Could you check a few things on this model? Use its own coordinates, in mm. Coordinates: 2 decimals unless noted, no trailing zeros. Loops run counter-clockwise (first coordinate to the right, second up) from the corner with the lowest first, then second, coordinate; pieces in that order, holes last.
1) Imagine slicing it at D-D on z = 0.4. Give the number of separate pieces and of enclosed holes in the cut face, plus the area to 3 significant figures.
2) Imagine slicing it at B-B on y = 26. Please give me the cut outline in (x, z).
3) Imagine slicing it at C-C on x = 5. Please give me the cut outline in (y, z).
4) Imagine slicing it at A-A on x = 32. Please give me the cut outline in (y, z).
5) If I drill on line 1 along X through (y, z) = (-3, 0.75); line 2 along Y through (x, z) = (-18, 0.9); line 3 along Y through (x, z) = (4, 0.25), over which ranges is the centre line in solid material (lowest first)?
6) Will these pins go through, and if not, where does the flat tip stop? P1, Ø0.6, axis at x = 22.5, z = 1, coming from the -Y side; P2, Ø0.6, axis at x = 17.5, z = 1.5, coming from the +Y side; P3, Ø1, axis at x = 17.5, z = 1.5, coming from the -Y side; P4, Ø3.5, axis at x = 32.63, y = 15.21, coming from the +Z side.
```python
from build123d import *

# Parameters (mm, degrees)
SKETCH1_R                = 40
SKETCH1_R_2              = 35
BOSS_EXTRUDE1_DEPTH      = 2
BOSS_EXTRUDE2_DEPTH      = 2
SKETCH3_R                = 3
CUT_EXTRUDE1_DEPTH       = 2
FILLET1_DEPTH            = 2
SKETCH4_R                = 2
CUT_EXTRUDE2_DEPTH       = 10
BOSS_EXTRUDE3_START      = -2
BOSS_EXTRUDE3_DEPTH      = 2
BOSS_EXTRUDE4_START      = -2
SKETCH7_R                = 13.5
SKETCH7_R_2              = 10.5
BOSS_EXTRUDE4_DEPTH      = 2
FILLET2_R                = 6
CUT_EXTRUDE3_DEPTH       = 3
CIRPATTERN1_COUNT        = 3
FILLET2_OF_CIRPATTERN1_R = 6
FILLET3_R                = 6


with BuildPart() as part:
    # Sketch1 → Boss-Extrude1 (new body)
    with BuildSketch(Plane.XY):
        Circle(SKETCH1_R)
        Circle(SKETCH1_R_2, mode=Mode.SUBTRACT)
    extrude(amount=BOSS_EXTRUDE1_DEPTH)

    # Sketch2 → Boss-Extrude2 (add)
    with BuildSketch(Plane(origin=(0, 0, 0), x_dir=(-1, 0, 0), z_dir=(0, 0, -1))):
        with BuildLine():
            Line((-29, 5), (-34.641016151, 5))
            Line((-34.641016151, 5), (-37.165171868, 5))
            ThreePointArc((-37.165171868, 5), (-37.5, 0), (-37.165171868, -5))
            Line((-37.165171868, -5), (-29, -5))
            ThreePointArc((-29, -5), (-24, 0), (-29, 5))
        make_face()
        with BuildLine():
            Line((-34, -3), (-29, -3))
            ThreePointArc((-29, -3), (-26, 0), (-29, 3))
            Line((-29, 3), (-34, 3))
            ThreePointArc((-34, 3), (-37, 0), (-34, -3))
        make_face(mode=Mode.SUBTRACT)
    boss_extrude2 = extrude(amount=-BOSS_EXTRUDE2_DEPTH)

    # Sketch3 → Cut-Extrude1 (cut)
    with BuildSketch(Plane(origin=(0, 0, 0), x_dir=(-1, 0, 0), z_dir=(0, 0, -1))):
        with Locations((-34, 0)):
            Circle(SKETCH3_R)
    cut_extrude1 = extrude(amount=-CUT_EXTRUDE1_DEPTH, mode=Mode.SUBTRACT)

    # Fillet1: read off the stored shape, not the designer's step
    # Fillet1 outline → Fillet1 (add)
    with BuildSketch(Plane.XY):
        with BuildLine():
            ThreePointArc((29, -5), (26.543386825, -4.354888254), (24.720689655, -2.586020683))
            ThreePointArc((24.720689655, -2.586020683), (26.992450638, -17.835874241), (17.74137931, -30.170241301))
            ThreePointArc((17.74137931, -30.170241301), (29.057943842, -19.509892353), (34.641016151, -5))
            Line((34.641016151, -5), (29, -5))
        make_face()
        with BuildLine():
            ThreePointArc((17.74137931, 30.170241301), (26.992450638, 17.835874241), (24.720689655, 2.586020683))
            ThreePointArc((24.720689655, 2.586020683), (26.543386825, 4.354888254), (29, 5))
            Line((29, 5), (34.641016151, 5))
            ThreePointArc((34.641016151, 5), (29.057943842, 19.509892353), (17.74137931, 30.170241301))
        make_face()
    fillet1 = extrude(amount=FILLET1_DEPTH)

    # Sketch4 → Cut-Extrude2 (cut)
    with BuildSketch(Plane.XY.offset(2)):
        with Locations((32.627080333, 15.214257423)):
            Circle(SKETCH4_R)
    cut_extrude2 = extrude(amount=-CUT_EXTRUDE2_DEPTH, mode=Mode.SUBTRACT)

    # Sketch5 → Boss-Extrude3 (add)
    with BuildSketch(Plane.XY.offset(2).offset(BOSS_EXTRUDE3_START)):
        with BuildLine():
            Line((7.348469228, 7.5), (34.186985828, 7.5))
            ThreePointArc((34.186985828, 7.5), (34.60231879, 5.261134323), (34.871191548, 3))
            Line((34.871191548, 3), (29, 3))
            ThreePointArc((29, 3), (26, 0), (29, -3))
            Line((29, -3), (34.871191548, -3))
            ThreePointArc((34.871191548, -3), (34.60231879, -5.261134323), (34.186985828, -7.5))
            Line((34.186985828, -7.5), (7.348469228, -7.5))
            ThreePointArc((7.348469228, -7.5), (10.5, 0), (7.348469228, 7.5))
        make_face()
    boss_extrude3 = extrude(amount=BOSS_EXTRUDE3_DEPTH)

    # Sketch7 → Boss-Extrude4 (add)
    with BuildSketch(Plane.XY.offset(2).offset(BOSS_EXTRUDE4_START)):
        Circle(SKETCH7_R)
        with Locations(Location((0, 0, 0), (0, 0, 180))):
            Circle(SKETCH7_R_2, mode=Mode.SUBTRACT)
    extrude(amount=BOSS_EXTRUDE4_DEPTH)

    # Fillet2
    fillet2_edges = [part.edges().sort_by_distance(p)[0] for p in [
        (11.22497216, 7.5, 1),
        (11.22497216, -7.5, 1),
        (26.852187894, 7.5, 1),
        (26.852187894, -7.5, 1),
    ]]
    fillet(fillet2_edges, radius=FILLET2_R)

    # Sketch6 → Cut-Extrude3 (cut)
    with BuildSketch(Plane.XY.offset(2)):
        with BuildLine():
            Line((0, 5), (34, 5))
            ThreePointArc((34, 5), (39, 0), (34, -5))
            Line((34, -5), (0, -5))
            Line((0, -5), (0, 5))
        make_face()
    cut_extrude3 = extrude(amount=-CUT_EXTRUDE3_DEPTH, mode=Mode.SUBTRACT)

    # CirPattern1: Boss-Extrude2, Cut-Extrude1, Fillet1, Cut-Extrude2, Boss-Extrude3, Cut-Extrude3 ×3 about axis
    cirpattern1_axis = Axis((0, 0, 0), (0, 0, 1))
    add([boss_extrude2.rotate(cirpattern1_axis, i * 360 / CIRPATTERN1_COUNT) for i in range(1, CIRPATTERN1_COUNT)])
    add([cut_extrude1.rotate(cirpattern1_axis, i * 360 / CIRPATTERN1_COUNT) for i in range(1, CIRPATTERN1_COUNT)], mode=Mode.SUBTRACT)
    add([fillet1.rotate(cirpattern1_axis, i * 360 / CIRPATTERN1_COUNT) for i in range(1, CIRPATTERN1_COUNT)])
    add([cut_extrude2.rotate(cirpattern1_axis, i * 360 / CIRPATTERN1_COUNT) for i in range(1, CIRPATTERN1_COUNT)], mode=Mode.SUBTRACT)
    add([boss_extrude3.rotate(cirpattern1_axis, i * 360 / CIRPATTERN1_COUNT) for i in range(1, CIRPATTERN1_COUNT)])
    add([cut_extrude3.rotate(cirpattern1_axis, i * 360 / CIRPATTERN1_COUNT) for i in range(1, CIRPATTERN1_COUNT)], mode=Mode.SUBTRACT)

    # Fillet2 of CirPattern1
    fillet2_of_cirpattern1_edges = [part.edges().sort_by_distance(p)[0] for p in [
        (-12.107676609, 5.971111048, 1),
        (0.882704448, 13.471111048, 1),
        (-19.921284476, 19.504676864, 1),
        (-6.930903419, 27.004676864, 1),
        (0.882704448, -13.471111048, 1),
        (-12.107676609, -5.971111048, 1),
        (-6.930903419, -27.004676864, 1),
        (-19.921284476, -19.504676864, 1),
    ]]
    fillet(fillet2_of_cirpattern1_edges, radius=FILLET2_OF_CIRPATTERN1_R)

    # Fillet3
    fillet3_edges = [part.edges().sort_by_distance(p)[0] for p in [
        (9.233092656, -5, 1),
        (9.233092656, 5, 1),
        (-0.286419309, 10.496092796, 1),
        (-8.946673347, 5.496092796, 1),
        (-8.946673347, -5.496092796, 1),
        (-0.286419309, -10.496092796, 1),
    ]]
    fillet(fillet3_edges, radius=FILLET3_R)


solid = part.part
```
Filled in:
1. separate pieces: 1
1. enclosed holes: 7
1. area: 1,970 mm2
2. outline: (-30.4, 0) - (-20.78, 0) - (-20.78, 2) - (-30.4, 2) - close; (-9.24, 0) - (-5.08, 0) - (-5.08, 2) - (-9.24, 2) - close; (22.74, 0) - (30.4, 0) - (30.4, 2) - (22.74, 2) - close
3. outline: (-39.69, 0) - (-32.91, 0) - (-32.91, 2) - (-39.69, 2) - close; (-12.54, 0) - (-9.23, 0) - (-9.23, 2) - (-12.54, 2) - close; (9.23, 0) - (12.54, 0) - (12.54, 2) - (9.23, 2) - close; (32.91, 0) - (39.69, 0) - (39.69, 2) - (32.91, 2) - close
4. outline: (-24, 0) - (-5, 0) - (-5, 2) - (-24, 2) - close; (5, 0) - (13.32, 0) - (13.32, 2) - (5, 2) - close; (17.11, 0) - (24, 0) - (24, 2) - (17.11, 2) - close
5. line 1: x = -39.89 to -34.79, -13.16 to -10.06, 38 to 39.89
5. line 2: y = -35.72 to -34.34, -21.18 to -15.93, 15.93 to 21.18, 34.34 to 35.72
5. line 3: y = -39.8 to -32.76, -12.89 to -9.71, 9.71 to 12.89, 32.76 to 39.8
6. P1: stops at y = -33.27
6. P2: stops at y = 36.11
6. P3: stops at y = -36.21
6. P4: passes through
